Design review of the part built by this model. Coordinates are the model's own, in mm. Face numbers are marked on the shaded views. A direction names the side the tool comes from. Coordinates: 2 decimals unless noted, no trailing zeros. Write each loop counter-clockwise with the first axis right and the second up, starting at its lowest first coordinate (ties: lowest second). Pieces come first, ordered by that corner, then holes. Notation, with made-up numbers: (33, -17.75) -> (46, -17.75) arc R11 ccw to (46, -7.75) -> close; hole circle Ø2 at (8.5, -33.75). An arc over 180 degrees is marked (long way). One line per question, with ' | ' between items. Start each with the question number.
Q1. Add section A-A on z = 23. State the section outline as (x, y) points, and give its area (3 significant figures).
Q2. For P1, Ø9.5, axis at x = 0, y = 0, coming from the -Z side; P2, Ø3, axis at x = -2, y = 20.5, coming from the +Z side; P3, Ø10, axis at x = -20.5, z = 11.5, coming from the +Y side; P4, Ø11.5, axis at x = 4, y = 2.5, coming from the -Z side, all flat-tipped, find the tip position at first contact; note any pin that passes through.
Q3. Draft analysis for pull direction X (two halves, no side actions). For the marked faces 1, 2 and 3, state which applies: pulls with the +X half, pulls with the -X half, needs draft (parallel to the pull), parting line crosses it, or undercut.
Q4. For the marked faces 4 and 5, list the 3-axis set-ups (+Z, -Z, +X, -X, +Y, -Y) from which the entire face can be reached by the end or side of a thin tool; tool diameter is ignored.
Q5. Add section B-B on z = 10. State the section outline as (x, y) points, and give its area (3 significant figures).
Q6. Wall thickness on probe 1 along Z at (x, y) = (32.5, 8.5); probe 2 along Y at (x, z) = (3.5, 24); probe 3 along Y at (x, z) = (0, 17.5) (3 decimals): over which ranges is each line inside the solid? List them lowest first.
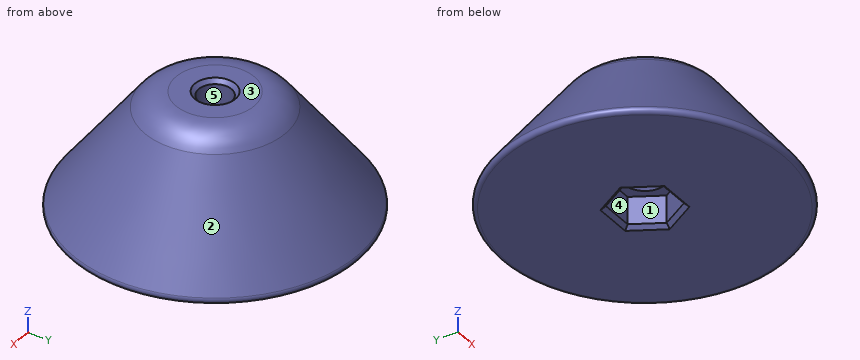
from build123d import *

# Parameters (mm, degrees)
FILLET1_R          = 1
FILLET2_R          = 10
SKETCH2_R          = 4.2
CUT_EXTRUDE1_DEPTH = 60.703433859
CUT_EXTRUDE2_START = -8
CUT_EXTRUDE2_DEPTH = 68.703433859
CHAMFER1_SIZE      = 1


with BuildPart() as part:
    # Sketch1 → Revolve1 (revolve)
    with BuildSketch(Plane(origin=(0, 0, 0), x_dir=(1, 0, 0), z_dir=(0, 1, 0))):
        Polygon((-37.5, 0), (0, 0), (0, -30), (-15, -30), align=None)
    revolve(axis=Axis((0, 0, 0), (0, 0, 1)))

    # Fillet1
    fillet1_edges = [part.edges().sort_by_distance(p)[0] for p in [
        (37.5, 0, 0),
    ]]
    fillet(fillet1_edges, radius=FILLET1_R)

    # Fillet2
    fillet2_edges = [part.edges().sort_by_distance(p)[0] for p in [
        (15, 0, 30),
    ]]
    fillet(fillet2_edges, radius=FILLET2_R)

    # Sketch2 → Cut-Extrude1 (cut, through all)
    with BuildSketch(Plane.XY.offset(30)):
        Circle(SKETCH2_R)
    extrude(amount=-CUT_EXTRUDE1_DEPTH, mode=Mode.SUBTRACT)

    # Sketch3 → Cut-Extrude2 (cut, through all)
    with BuildSketch(Plane(origin=(0, 0, 0), x_dir=(-1, 0, 0), z_dir=(0, 0, -1)).offset(CUT_EXTRUDE2_START)):
        Polygon((-8.29998747, 0), (-4.149993735, -7.188), (4.149993735, -7.188), (8.29998747, 0), (4.149993735, 7.188), (-4.149993735, 7.188), align=None)
    extrude(amount=CUT_EXTRUDE2_DEPTH, mode=Mode.SUBTRACT)

    # Chamfer1
    chamfer1_edges = [part.edges().sort_by_distance(p)[0] for p in [
        (-4.2, 0, 30),
        (6.224990602, 3.594, 0),
        (6.224990602, -3.594, 0),
        (0, -7.188, 0),
        (-6.224990602, -3.594, 0),
        (-6.224990602, 3.594, 0),
        (0, 7.188, 0),
        (-4.2, 0, 8),
    ]]
    chamfer(chamfer1_edges, length=CHAMFER1_SIZE)


solid = part.part
Output values:
1) outline: circle Ø40.5 at (0, 0); hole circle Ø8.4 at (0, 0) | area: 1,230 mm2
2) P1: stops at z = 8.45 | P2: stops at z = 24.54 | P3: stops at y = 26.64 | P4: stops at z = 0
3) face 1: undercut | face 2: parting line crosses it | face 3: needs draft
4) face 4: -Z | face 5: +Z, -Z
5) outline: circle Ø60 at (0, 0); hole circle Ø8.4 at (0, 0) | area: 2,770 mm2
6) probe 1: z = 0 to 5.21 | probe 2: y = -19.18 to -2.32, 2.32 to 19.18 | probe 3: y = -24.375 to -4.2, 4.2 to 24.375
